```python
from build123d import *

# Parameters (mm, degrees)
SKETCH1_W           = 1219.2
SKETCH1_H           = 1771.65
BOSS_EXTRUDE1_DEPTH = 9.525
SKETCH3_W           = 88.9
SKETCH3_H           = 76.2
SKETCH3_W_2         = 73.6727
CUT_EXTRUDE2_DEPTH  = 20.05
CHAMFER1_SIZE       = 2.54


with BuildPart() as part:
    # Sketch1 → Boss-Extrude1 (new body, symmetric)
    with BuildSketch(Plane(origin=(0, 0, 0), x_dir=(1, 0, 0), z_dir=(0, 1, 0))):
        with Locations((609.6, 885.825)):
            Rectangle(SKETCH1_W, SKETCH1_H)
    extrude(amount=BOSS_EXTRUDE1_DEPTH, both=True)

    # Sketch3 → Cut-Extrude2 (cut, through all)
    with BuildSketch(Plane(origin=(0, 9.525, 0), x_dir=(1, 0, 0), z_dir=(0, 1, 0))):
        with Locations((44.45, 1733.55)):
            Rectangle(SKETCH3_W, SKETCH3_H)
        with Locations((254.6477, 1733.55)):
            Rectangle(SKETCH3_W, SKETCH3_H)
        with Locations((750.9256, 646.112499999)):
            Rectangle(SKETCH3_W, SKETCH3_H)
        with Locations((44.45, 38.1)):
            Rectangle(SKETCH3_W, SKETCH3_H)
        with Locations((750.9256, 38.1)):
            Rectangle(SKETCH3_W, SKETCH3_H)
        with Locations((1182.36365, 1733.55)):
            Rectangle(SKETCH3_W_2, SKETCH3_H)
    extrude(amount=-CUT_EXTRUDE2_DEPTH, mode=Mode.SUBTRACT)

    # Chamfer1
    chamfer1_edges = [part.edges().sort_by_distance(p)[0] for p in [
        (1219.2, 9.525, -847.725),
        (0, 9.525, -885.825),
        (397.6878, 9.525, 0),
        (1007.2878, 9.525, 0),
        (722.3125, 9.525, -1771.65),
        (149.54885, 9.525, -1771.65),
        (1145.5273, 9.525, -1733.55),
        (1182.36365, 9.525, -1695.45),
        (795.3756, 9.525, -38.1),
        (750.9256, 9.525, -76.2),
        (706.4756, 9.525, -38.1),
        (88.9, 9.525, -38.1),
        (44.45, 9.525, -76.2),
        (706.4756, 9.525, -646.112499999),
        (750.9256, 9.525, -608.012499999),
        (795.3756, 9.525, -646.112499999),
        (750.9256, 9.525, -684.212499999),
        (210.1977, 9.525, -1733.55),
        (254.6477, 9.525, -1695.45),
        (299.0977, 9.525, -1733.55),
        (44.45, 9.525, -1695.45),
        (88.9, 9.525, -1733.55),
    ]]
    chamfer(chamfer1_edges, length=CHAMFER1_SIZE)


solid = part.part
```
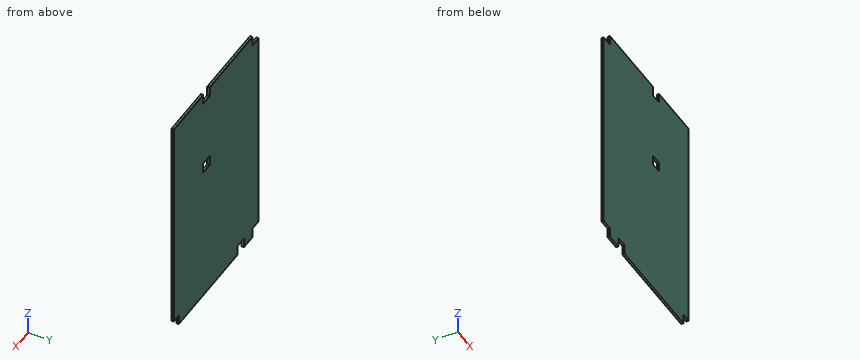
Can you work these out from the model? Positions are in its coordinate system, mm. Give positions to 0.01 mm unless a question says otherwise; leave off trailing zeros. Order: outer loops, then holes, each group sorted by start corner. A loop starts at its lowest first (then second) coordinate and runs counter-clockwise, first axis right, second up. Notation, with made-up numbers: (35, 52.25) - (89, 52.25) arc R24 cw to (89, 64.25) - close; hole circle Ø6 at (62.5, 86). An arc over 180 degrees is marked (long way). Use a Markdown table: item, result. Add a question column.
Q1. If we section it at A-A on z = -664: Write out the boundary of the cut face in (x, y) (3 decimals), plus the area to 3 significant figures.
Q2. I'm going to push flat-ended pins straight in: pin 1 (8.5 mm diameter, centred on x = 42.5, y = 1, fed in from -Z); pin 2 (8.5 mm diameter, centred on y = -4.5, z = -1735, fed in from -X); pin 3 (8.5 mm diameter, centred on y = -1, z = -1714.5, fed in from +X). Where does each tip first touch, or does it pass through?
Q3. Please list where these lines run through material, in increasing order: line 1 along Z through (x, y) = (1161.5, 3.5); line 2 along X through (y, z) = (7.75, -1028) (3 decimals); line 3 along Z through (x, y) = (693.5, 7.5) (3 decimals).
Q4. If we section it at B-B on y = 1: Write out the boundary of the cut face in (x, z), plus the area to 3 significant figures.
Q5. If we section it at D-D on x = 259: Write out the boundary of the cut face in (y, z) (3 decimals), plus the area to 3 significant figures.
Answers follow:
| question | item | result |
|---|---|---|
| 1 | outline | (0, -9.525) - (706.476, -9.525) - (706.476, 6.985) - (703.936, 9.525) - (2.54, 9.525) - (0, 6.985) - close; (795.376, -9.525) - (1219.2, -9.525) - (1219.2, 6.985) - (1216.66, 9.525) - (797.916, 9.525) - (795.376, 6.985) - close |
| 1 | area | 21,500 mm^2 |
| 2 | pin 1 | stops at z = -1695.45 |
| 2 | pin 2 | stops at x = 88.9 |
| 2 | pin 3 | stops at x = 1145.53 |
| 3 | line 1 | z = -1695.45 to 0 |
| 3 | line 2 | x = 0.765 to 1218.435 |
| 3 | line 3 | z = -1771.135 to -0.515 |
| 4 | outline | (0, -1695.45) - (88.9, -1695.45) - (88.9, -1771.65) - (210.2, -1771.65) - (210.2, -1695.45) - (299.1, -1695.45) - (299.1, -1771.65) - (1145.53, -1771.65) - (1145.53, -1695.45) - (1219.2, -1695.45) - (1219.2, 0) - (795.38, 0) - (795.38, -76.2) - (706.48, -76.2) - (706.48, 0) - (88.9, 0) - (88.9, -76.2) - (0, -76.2) - close; hole (706.48, -684.21) - (795.38, -684.21) - (795.38, -608.01) - (706.48, -608.01) - close |
| 4 | area | 2,120,000 mm^2 |
| 5 | outline | (-9.525, -1695.45) - (6.985, -1695.45) - (9.525, -1692.91) - (9.525, -2.54) - (6.985, 0) - (-9.525, 0) - close |
| 5 | area | 32,300 mm^2 |
